For this review, take the finished solid that the model builds, in its own axes (mm). Coordinates: 2 decimals unless noted, no trailing zeros. Loops run counter-clockwise (first coordinate to the right, second up) from the corner with the lowest first, then second, coordinate; pieces in that order, holes last. Notation, with made-up numbers: (13, 51) - (60, 51) arc R30 ccw to (60, 83) - close; hole circle Ø8 at (23, 35). An arc over 180 degrees is marked (long way). Answer as a JSON object with one key per item and string values. Group by question number.
Item 1: We need section C-C (z = -50). Give the boundary of the cut face in (x, y), then the cut area to 3 significant figures.
Item 2: Clearance check with flat-ended pins moving along their axes: pin 1 (3 mm diameter, centred on x = -54.5, y = 3, fed in from -Z); pin 2 (1.6 mm diameter, centred on x = -0.5, y = 4.5, fed in from -Z); pin 3 (3 mm diameter, centred on y = 3, z = -9.5, fed in from +X). State where each tip first meets the part, or that it passes through.
Item 3: To check wall thickness, follow line 1 (X direction, y = 1.9, z = 0); line 2 (X direction, y = 9.75, z = 2); line 3 (Z direction, x = 38, y = 2). State the ranges of each line that lie inside material, in increasing order.
Item 4: We need section B-B (x = -32). Give the boundary of the cut face in (y, z), then the cut area to 3 significant figures.
Item 5: We need section A-A (z = 23). Give the boundary of the cut face in (x, y), then the cut area to 3 significant figures.
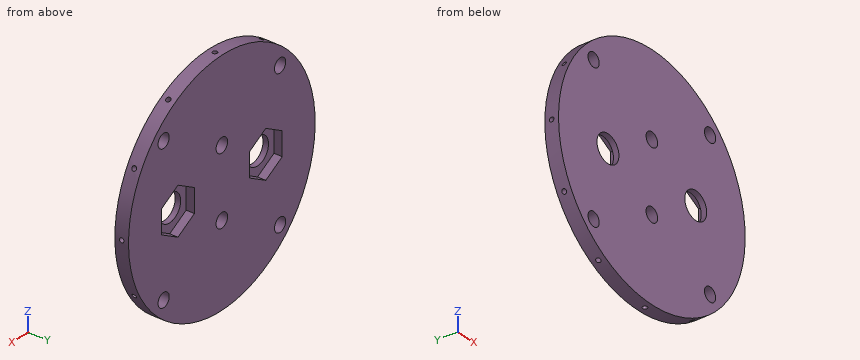
from build123d import *

# Parameters (mm, degrees)
SZKIC1_R                    = 85
DODANIE_WYCI_GNI_CIE1_DEPTH = 10
CUT_EXTRUDE1_REACH          = 122.623
SZKIC2_R                    = 10
SZKIC2_R_2                  = 5.25
SZKIC2_R_3                  = 5.1
CUT_EXTRUDE2_DEPTH          = 6
SKETCH2_R                   = 1.65
CUT_EXTRUDE3_DEPTH          = 12
CIRPATTERN1_COUNT           = 12


with BuildPart() as part:
    # Szkic1 → Dodanie-wyciągnięcie1 (new body)
    with BuildSketch(Plane(origin=(0, 0, 0), x_dir=(1, 0, 0), z_dir=(0, 1, 0))):
        with Locations(Location((0, 0, 0), (0, 0, 270))):
            Circle(SZKIC1_R)
    extrude(amount=DODANIE_WYCI_GNI_CIE1_DEPTH)

    # Szkic2 → Cut-Extrude1 (cut, up to next)
    with BuildSketch(Plane(origin=(0, 10, 0), x_dir=(1, 0, 0), z_dir=(0, 1, 0)), mode=Mode.PRIVATE) as cut_extrude1_sk1:
        with Locations(Location((-40, 0, 0), (0, 0, 270))):
            Circle(SZKIC2_R)
    cut_extrude1_tool1 = extrude(cut_extrude1_sk1.sketch, amount=-CUT_EXTRUDE1_REACH, mode=Mode.PRIVATE) & part.part
    # Szkic2 → Cut-Extrude1 (cut, up to next)
    with BuildSketch(Plane(origin=(0, 10, 0), x_dir=(1, 0, 0), z_dir=(0, 1, 0)), mode=Mode.PRIVATE) as cut_extrude1_sk2:
        with Locations(Location((0, 25, 0), (0, 0, 270))):
            Circle(SZKIC2_R_2)
    cut_extrude1_tool2 = extrude(cut_extrude1_sk2.sketch, amount=-CUT_EXTRUDE1_REACH, mode=Mode.PRIVATE) & part.part
    # Szkic2 → Cut-Extrude1 (cut, up to next)
    with BuildSketch(Plane(origin=(0, 10, 0), x_dir=(1, 0, 0), z_dir=(0, 1, 0)), mode=Mode.PRIVATE) as cut_extrude1_sk3:
        with Locations(Location((53.033008589, 53.033008589, 0), (0, 0, 270))):
            Circle(SZKIC2_R_3)
    cut_extrude1_tool3 = extrude(cut_extrude1_sk3.sketch, amount=-CUT_EXTRUDE1_REACH, mode=Mode.PRIVATE) & part.part
    # Szkic2 → Cut-Extrude1 (cut, up to next)
    with BuildSketch(Plane(origin=(0, 10, 0), x_dir=(1, 0, 0), z_dir=(0, 1, 0)), mode=Mode.PRIVATE) as cut_extrude1_sk4:
        with Locations(Location((53.033008589, -53.033008589, 0), (0, 0, 270))):
            Circle(SZKIC2_R_3)
    cut_extrude1_tool4 = extrude(cut_extrude1_sk4.sketch, amount=-CUT_EXTRUDE1_REACH, mode=Mode.PRIVATE) & part.part
    # Szkic2 → Cut-Extrude1 (cut, up to next)
    with BuildSketch(Plane(origin=(0, 10, 0), x_dir=(1, 0, 0), z_dir=(0, 1, 0)), mode=Mode.PRIVATE) as cut_extrude1_sk5:
        with Locations(Location((-53.033008589, -53.033008589, 0), (0, 0, 270))):
            Circle(SZKIC2_R_3)
    cut_extrude1_tool5 = extrude(cut_extrude1_sk5.sketch, amount=-CUT_EXTRUDE1_REACH, mode=Mode.PRIVATE) & part.part
    # Szkic2 → Cut-Extrude1 (cut, up to next)
    with BuildSketch(Plane(origin=(0, 10, 0), x_dir=(1, 0, 0), z_dir=(0, 1, 0)), mode=Mode.PRIVATE) as cut_extrude1_sk6:
        with Locations(Location((-53.033008589, 53.033008589, 0), (0, 0, 270))):
            Circle(SZKIC2_R_3)
    cut_extrude1_tool6 = extrude(cut_extrude1_sk6.sketch, amount=-CUT_EXTRUDE1_REACH, mode=Mode.PRIVATE) & part.part
    # Szkic2 → Cut-Extrude1 (cut, up to next)
    with BuildSketch(Plane(origin=(0, 10, 0), x_dir=(1, 0, 0), z_dir=(0, 1, 0)), mode=Mode.PRIVATE) as cut_extrude1_sk7:
        with Locations(Location((0, -25, 0), (0, 0, 270))):
            Circle(SZKIC2_R_2)
    cut_extrude1_tool7 = extrude(cut_extrude1_sk7.sketch, amount=-CUT_EXTRUDE1_REACH, mode=Mode.PRIVATE) & part.part
    # Szkic2 → Cut-Extrude1 (cut, up to next)
    with BuildSketch(Plane(origin=(0, 10, 0), x_dir=(1, 0, 0), z_dir=(0, 1, 0)), mode=Mode.PRIVATE) as cut_extrude1_sk8:
        with Locations(Location((40, 0, 0), (0, 0, 270))):
            Circle(SZKIC2_R)
    cut_extrude1_tool8 = extrude(cut_extrude1_sk8.sketch, amount=-CUT_EXTRUDE1_REACH, mode=Mode.PRIVATE) & part.part
    add(cut_extrude1_tool1.solids().sort_by_distance((-40, 10, 0))[0], mode=Mode.SUBTRACT)
    add(cut_extrude1_tool2.solids().sort_by_distance((0, 10, -25))[0], mode=Mode.SUBTRACT)
    add(cut_extrude1_tool3.solids().sort_by_distance((53.033009, 10, -53.033009))[0], mode=Mode.SUBTRACT)
    add(cut_extrude1_tool4.solids().sort_by_distance((53.033009, 10, 53.033009))[0], mode=Mode.SUBTRACT)
    add(cut_extrude1_tool5.solids().sort_by_distance((-53.033009, 10, 53.033009))[0], mode=Mode.SUBTRACT)
    add(cut_extrude1_tool6.solids().sort_by_distance((-53.033009, 10, -53.033009))[0], mode=Mode.SUBTRACT)
    add(cut_extrude1_tool7.solids().sort_by_distance((0, 10, 25))[0], mode=Mode.SUBTRACT)
    add(cut_extrude1_tool8.solids().sort_by_distance((40, 10, 0))[0], mode=Mode.SUBTRACT)

    # Sketch1 → Cut-Extrude2 (cut)
    with BuildSketch(Plane(origin=(0, 10, 0), x_dir=(1, 0, 0), z_dir=(0, 1, 0))):
        Polygon((-25, -8.660254038), (-25, 8.660254038), (-40, 17.320508076), (-55, 8.660254038), (-55, -8.660254038), (-40, -17.320508076), align=None)
        Polygon((25, -8.660254038), (40, -17.320508076), (55, -8.660254038), (55, 8.660254038), (40, 17.320508076), (25, 8.660254038), align=None)
    extrude(amount=-CUT_EXTRUDE2_DEPTH, mode=Mode.SUBTRACT)

    # Sketch2 → Cut-Extrude3 (cut)
    with BuildSketch(Plane.ZY.offset(85)):
        with Locations((0, 5)):
            Circle(SKETCH2_R)
    cut_extrude3 = extrude(amount=-CUT_EXTRUDE3_DEPTH, mode=Mode.SUBTRACT)

    # CirPattern1: Cut-Extrude3 ×12 about axis
    cirpattern1_axis = Axis((0, 0, 0), (0, 1, 0))
    for i in range(1, CIRPATTERN1_COUNT):
        add(cut_extrude3.rotate(cirpattern1_axis, i * 360 / CIRPATTERN1_COUNT), mode=Mode.SUBTRACT)


solid = part.part
Check sheet entries:
{
 "1": {"outline": "(-68.74, 0) - (-57.13, 0) - (-57.13, 10) - (-68.74, 10) - close; (-48.93, 0) - (48.93, 0) - (48.93, 10) - (-48.93, 10) - close; (57.13, 0) - (68.74, 0) - (68.74, 10) - (57.13, 10) - close", "area": "1,210 mm2"},
 "2": {"pin 1": "stops at z = -66.45", "pin 2": "stops at z = -73", "pin 3": "stops at x = 84.62"},
 "3": {"line 1": "x = -85 to -50, -30 to 30, 50 to 85", "line 2": "x = -84.98 to -55, -25 to 25, 55 to 84.98", "line 3": "z = -76.03 to -9.8, 9.8 to 76.03"},
 "4": {"outline": "(0, -78.75) - (10, -78.75) - (10, -12.7) - (4, -12.7) - (4, -6) - (0, -6) - close; (0, 6) - (4, 6) - (4, 12.7) - (10, 12.7) - (10, 78.75) - (0, 78.75) - close", "area": "1,370 mm2"},
 "5": {"outline": "(-81.83, 0) - (-4.85, 0) - (-4.85, 10) - (-81.83, 10) - close; (4.85, 0) - (81.83, 0) - (81.83, 10) - (4.85, 10) - close", "area": "1,540 mm2"}
}
